CAD build for the part. Positions are in the model's coordinates, mm. Face numbers are marked on the shaded views. A direction names the side the tool comes from. Round coordinates to 2 decimals unless told otherwise and drop trailing zeros. Write each loop counter-clockwise with the first axis right and the second up, starting at its lowest first coordinate (ties: lowest second). Pieces come first, ordered by that corner, then holes. Notation, with made-up numbers: (-27, 7.5) -> (10, 7.5) arc R29 cw to (10, 43.5) -> close; hole circle Ø2 at (-27, 66.5). An arc over 180 degrees is marked (long way). Answer in a Markdown table with one row per item. Add a question column.
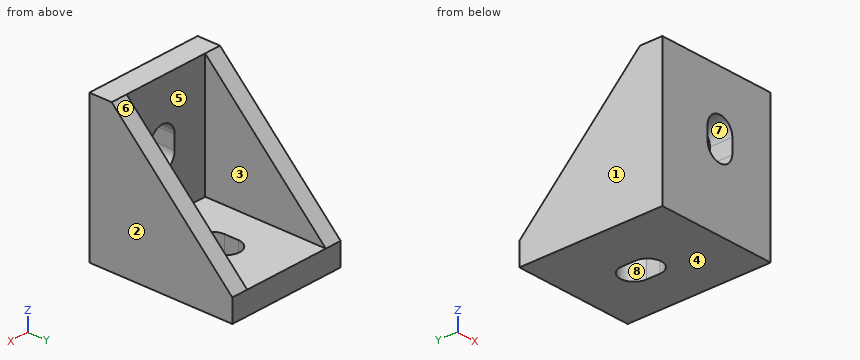
```python
from build123d import *

# Parameters (mm, degrees)
SKETCH1_W           = 16.7005
SKETCH1_H           = 19.9898
BOSS_EXTRUDE1_DEPTH = 3.1242
SKETCH3_W           = 16.7005
SKETCH3_H           = 3.1242
BOSS_EXTRUDE2_DEPTH = 19.9898
BOSS_EXTRUDE3_DEPTH = 2.286
BOSS_EXTRUDE4_DEPTH = 2.286
CUT_EXTRUDE1_REACH  = 29.455
SKETCH6_R           = 1.905
CUT_EXTRUDE2_START  = -3.1242
CUT_EXTRUDE2_DEPTH  = 3.1242


# Read off the part's stored shape, not the designer's step: Cut-Extrude2
with BuildPart() as part:
    # Sketch1 → Boss-Extrude1 (new body)
    with BuildSketch(Plane(origin=(0, 0, 0), x_dir=(1, 0, 0), z_dir=(0, 1, 0))):
        Rectangle(SKETCH1_W, SKETCH1_H)
    extrude(amount=BOSS_EXTRUDE1_DEPTH)

    # Sketch3 → Boss-Extrude2 (add)
    with BuildSketch(Plane.XZ):
        with Locations((0, -8.4328)):
            Rectangle(SKETCH3_W, SKETCH3_H)
    extrude(amount=-BOSS_EXTRUDE2_DEPTH)

    # Sketch4 → Boss-Extrude3 (add)
    with BuildSketch(Plane(origin=(8.35025, 0, 0), x_dir=(0, 0, -1), z_dir=(1, 0, 0))):
        Polygon((6.8707, 19.9898), (-9.9949, 3.1242), (6.8707, 3.1242), align=None)
    extrude(amount=-BOSS_EXTRUDE3_DEPTH)

    # Sketch5 → Boss-Extrude4 (add)
    with BuildSketch(Plane.ZY.offset(8.35025)):
        Polygon((-6.8707, 19.9898), (9.9949, 3.1242), (-6.8707, 3.1242), align=None)
    extrude(amount=-BOSS_EXTRUDE4_DEPTH)

    # Sketch6 → Cut-Extrude1 (cut, up to next)
    with BuildSketch(Plane.XY.offset(-6.8707), mode=Mode.PRIVATE) as cut_extrude1_sk1:
        with Locations((0.53975, 10.1092)):
            Circle(SKETCH6_R)
    cut_extrude1_tool1 = extrude(cut_extrude1_sk1.sketch, amount=-CUT_EXTRUDE1_REACH, mode=Mode.PRIVATE) & part.part
    # Sketch6 → Cut-Extrude1 (cut, up to next)
    with BuildSketch(Plane.XY.offset(-6.8707), mode=Mode.PRIVATE) as cut_extrude1_sk2:
        with Locations((0.53975, 12.0142)):
            Circle(SKETCH6_R)
    cut_extrude1_tool2 = extrude(cut_extrude1_sk2.sketch, amount=-CUT_EXTRUDE1_REACH, mode=Mode.PRIVATE) & part.part
    # Sketch6 → Cut-Extrude1 (cut, up to next)
    with BuildSketch(Plane.XY.offset(-6.8707), mode=Mode.PRIVATE) as cut_extrude1_sk3:
        with BuildLine():
            Line((2.44475, 10.1092), (2.44475, 12.0142))
            ThreePointArc((2.44475, 12.0142), (2.379838699, 11.521149719), (2.189528394, 11.0617))
            ThreePointArc((2.189528394, 11.0617), (2.379838699, 10.602250281), (2.44475, 10.1092))
        make_face()
    cut_extrude1_tool3 = extrude(cut_extrude1_sk3.sketch, amount=-CUT_EXTRUDE1_REACH, mode=Mode.PRIVATE) & part.part
    # Sketch6 → Cut-Extrude1 (cut, up to next)
    with BuildSketch(Plane.XY.offset(-6.8707), mode=Mode.PRIVATE) as cut_extrude1_sk4:
        with Locations((0.53975, 12.0142)):
            Circle(SKETCH6_R)
    cut_extrude1_tool4 = extrude(cut_extrude1_sk4.sketch, amount=-CUT_EXTRUDE1_REACH, mode=Mode.PRIVATE) & part.part
    # Sketch6 → Cut-Extrude1 (cut, up to next)
    with BuildSketch(Plane.XY.offset(-6.8707), mode=Mode.PRIVATE) as cut_extrude1_sk5:
        with Locations((0.53975, 10.1092)):
            Circle(SKETCH6_R)
    cut_extrude1_tool5 = extrude(cut_extrude1_sk5.sketch, amount=-CUT_EXTRUDE1_REACH, mode=Mode.PRIVATE) & part.part
    # Sketch6 → Cut-Extrude1 (cut, up to next)
    with BuildSketch(Plane.XY.offset(-6.8707), mode=Mode.PRIVATE) as cut_extrude1_sk6:
        with BuildLine():
            ThreePointArc((-1.110028394, 11.0617), (-1.300338699, 11.521149719), (-1.36525, 12.0142))
            Line((-1.36525, 12.0142), (-1.36525, 10.1092))
            ThreePointArc((-1.36525, 10.1092), (-1.300338699, 10.602250281), (-1.110028394, 11.0617))
        make_face()
    cut_extrude1_tool6 = extrude(cut_extrude1_sk6.sketch, amount=-CUT_EXTRUDE1_REACH, mode=Mode.PRIVATE) & part.part
    # Sketch6 → Cut-Extrude1 (cut, up to next)
    with BuildSketch(Plane.XY.offset(-6.8707), mode=Mode.PRIVATE) as cut_extrude1_sk7:
        with Locations((0.53975, 10.1092)):
            Circle(SKETCH6_R)
    cut_extrude1_tool7 = extrude(cut_extrude1_sk7.sketch, amount=-CUT_EXTRUDE1_REACH, mode=Mode.PRIVATE) & part.part
    # Sketch6 → Cut-Extrude1 (cut, up to next)
    with BuildSketch(Plane.XY.offset(-6.8707), mode=Mode.PRIVATE) as cut_extrude1_sk8:
        with Locations((0.53975, 12.0142)):
            Circle(SKETCH6_R)
    cut_extrude1_tool8 = extrude(cut_extrude1_sk8.sketch, amount=-CUT_EXTRUDE1_REACH, mode=Mode.PRIVATE) & part.part
    add(cut_extrude1_tool1.solids().sort_by_distance((0.53975, 10.1092, -6.8707))[0], mode=Mode.SUBTRACT)
    add(cut_extrude1_tool2.solids().sort_by_distance((0.53975, 12.0142, -6.8707))[0], mode=Mode.SUBTRACT)
    add(cut_extrude1_tool3.solids().sort_by_distance((2.369151, 11.0617, -6.8707))[0], mode=Mode.SUBTRACT)
    add(cut_extrude1_tool4.solids().sort_by_distance((0.53975, 12.0142, -6.8707))[0], mode=Mode.SUBTRACT)
    add(cut_extrude1_tool5.solids().sort_by_distance((0.53975, 10.1092, -6.8707))[0], mode=Mode.SUBTRACT)
    add(cut_extrude1_tool6.solids().sort_by_distance((-1.289651, 11.0617, -6.8707))[0], mode=Mode.SUBTRACT)
    add(cut_extrude1_tool7.solids().sort_by_distance((0.53975, 10.1092, -6.8707))[0], mode=Mode.SUBTRACT)
    add(cut_extrude1_tool8.solids().sort_by_distance((0.53975, 12.0142, -6.8707))[0], mode=Mode.SUBTRACT)

    # Cut-Extrude2 outline → Cut-Extrude2 (cut)
    with BuildSketch(Plane(origin=(0, 3.1242, 0), x_dir=(1, 0, 0), z_dir=(0, 1, 0)).offset(CUT_EXTRUDE2_START)):
        with BuildLine():
            Line((-1.36525, -0.4699), (-1.36525, -2.3749))
            ThreePointArc((-1.36525, -2.3749), (0.53975, -4.2799), (2.44475, -2.3749))
            Line((2.44475, -2.3749), (2.437778565, -0.307073202))
            ThreePointArc((2.437778565, -0.307073202), (0.458262015, 1.433356343), (-1.36525, -0.4699))
        make_face()
    extrude(amount=CUT_EXTRUDE2_DEPTH, mode=Mode.SUBTRACT)


solid = part.part
```
Item 1: Pin check, flat tips, straight feed: pin 1 (5 mm diameter, centred on x = 3.5, z = 8, fed in from -Y); pin 2 (2 mm diameter, centred on x = 0, y = 10.5, fed in from +Z); pin 3 (9.5 mm diameter, centred on x = 2.5, z = 1, fed in from +Y); pin 4 (3 mm diameter, centred on x = 6.5, z = -2.5, fed in from +Y). Stop position of each tip, or through.
Item 2: Saw through at B-B on x = 0. Give the cut face in (y, z), then the cut area to 3 significant figures.
Item 3: Drill centre lines: probe 1 along Z at (x, y) = (0.5, 2.75); probe 2 along X at (y, z) = (4, -3); probe 3 along Z at (x, y) = (5.25, 11.75). Where is each one in solid material? Low to high.
Item 4: Saw through at D-D on z = 1.5. Give the cut face in (x, y), then the cut area to 3 significant figures.
Item 5: Tool access for the marked faces 4, 5, 6, 7 and 8: list every direction of +Z, -Z, +X, -X, +Y, -Y with a clear straight run to the whole face (end or side of a thin tool).
Item 6: Two-plate mould, pull along X, no slides. Class the marked faces 1, 2 and 3: +X half, -X half, draft (parallel to the pull), parting line (faces both ways), or undercut.
Item 7: Saw through at A-A on z = -7.25. Give the cut face in (x, y) (3 decimals), then the cut area to 3 significant figures.
Item 8: Saw through at C-C on y = 10.75. Give the cut face in (x, z), then the cut area to 3 significant figures.
Recorded:
| question | item | result |
|---|---|---|
| 1 | pin 1 | y = 0 |
| 1 | pin 2 | through |
| 1 | pin 3 | y = 15.26 |
| 1 | pin 4 | y = 17.12 |
| 2 | outline | (0, -9.99) -> (8.28, -9.99) -> (8.28, -6.87) -> (3.12, -6.87) -> (3.12, -1.36) -> (0, -1.36) -> close; (0, 4.2) -> (3.12, 4.2) -> (3.12, 9.99) -> (0, 9.99) -> close; (13.84, -9.99) -> (19.99, -9.99) -> (19.99, -6.87) -> (13.84, -6.87) -> close |
| 2 | area | 80.4 mm2 |
| 3 | probe 1 | -9.99 to -1.43, 4.28 to 9.99 |
| 3 | probe 2 | -8.35 to -6.06, 6.06 to 8.35 |
| 3 | probe 3 | -9.99 to -6.87 |
| 4 | outline | (-8.35, 0) -> (-1.37, 0) -> (-1.37, 3.12) -> (-6.06, 3.12) -> (-6.06, 11.62) -> (-8.35, 11.62) -> close; (2.44, 0) -> (8.35, 0) -> (8.35, 11.62) -> (6.06, 11.62) -> (6.06, 3.12) -> (2.44, 3.12) -> close |
| 4 | area | 79.1 mm2 |
| 5 | face 4 | -Z, +X, -X, +Y, -Y |
| 5 | face 5 | +Z, +Y |
| 5 | face 6 | +Z, +X, -X, +Y |
| 5 | face 7 | +Y, -Y |
| 5 | face 8 | +Z, -Z |
| 6 | face 1 | -X half |
| 6 | face 2 | +X half |
| 6 | face 3 | undercut |
| 7 | outline | (-8.35, 0) -> (8.35, 0) -> (8.35, 19.99) -> (-8.35, 19.99) -> close; hole (-1.365, 10.109) arc R1.905 ccw to (2.445, 10.109) -> (2.445, 12.014) arc R1.905 ccw to (-1.365, 12.014) -> close |
| 7 | area | 315 mm2 |
| 8 | outline | (-8.35, -9.99) -> (-1.37, -9.99) -> (-1.37, -6.87) -> (-6.06, -6.87) -> (-6.06, 2.37) -> (-8.35, 2.37) -> close; (2.44, -9.99) -> (8.35, -9.99) -> (8.35, 2.37) -> (6.06, 2.37) -> (6.06, -6.87) -> (2.44, -6.87) -> close |
| 8 | area | 82.5 mm2 |
